Could you check a few things on this model? Use its own coordinates, in mm. A direction names the side the tool comes from. Coordinates: 2 decimals unless noted, no trailing zeros. Write each loop counter-clockwise with the first axis right and the second up, starting at its lowest first coordinate (ties: lowest second). Pieces come first, ordered by that corner, then holes.
```python
from build123d import *

# Parameters (mm, degrees)
F0_W      = 60
F0_H      = 15
F1_DEPTH  = 75
F2_DEPTH  = 15
F4_DEPTH  = 25
F6_DEPTH  = 40
F8_DEPTH  = 40
F10_DEPTH = 25


with BuildPart() as f1:
    # F0 (on Top) → F1 (new body)
    with BuildSketch(Plane.XY):
        with Locations((17.5909090042, 32.8136347234)):
            Rectangle(F0_W, F0_H)
    extrude(amount=F1_DEPTH)

    # F0 (on Top) → F2 (join)
    with BuildSketch(Plane.XY):
        with Locations((17.5909090042, 32.8136347234)):
            Rectangle(F0_W, F0_H)
        with BuildLine():
            Line((47.5909090042, 25.3136347234), (-12.4090909958, 25.3136347234))
            Line((-12.4090909958, 25.3136347234), (-12.4090909958, -29.6863652766))
            ThreePointArc((-12.4090909958, -29.6863652766), (17.5909090042, 0.3136347234), (47.5909090042, -29.6863652766))
            Line((47.5909090042, -29.6863652766), (47.5909090042, 25.3136347234))
        make_face()
        with BuildLine():
            ThreePointArc((47.5909090042, -29.6863652766), (17.5909090042, 0.3136347234), (-12.4090909958, -29.6863652766))
            Line((-12.4090909958, -29.6863652766), (47.5909090042, -29.6863652766))
        make_face()
        with BuildLine():
            Line((47.5909090042, -29.6863652766), (-12.4090909958, -29.6863652766))
            ThreePointArc((-12.4090909958, -29.6863652766), (17.5909090042, -59.6863652766), (47.5909090042, -29.6863652766))
        make_face()
    extrude(amount=F2_DEPTH)

    # F3 (on face) → F4 (cut)
    with BuildSketch(Plane.XY.offset(15)):
        with BuildLine():
            ThreePointArc((7.5909090042, -57.970636524), (17.5909090042, -59.6863652766), (27.5909090042, -57.970636524))
            Line((27.5909090042, -57.970636524), (27.5909090042, -29.6863652766))
            ThreePointArc((27.5909090042, -29.6863652766), (17.5909090042, -39.6863652766), (7.5909090042, -29.6863652766))
            Line((7.5909090042, -29.6863652766), (7.5909090042, -57.970636524))
        make_face()
        with BuildLine():
            ThreePointArc((7.5909090042, -29.6863652766), (17.5909090042, -39.6863652766), (27.5909090042, -29.6863652766))
            Line((27.5909090042, -29.6863652766), (17.5909090042, -29.6863652766))
            Line((17.5909090042, -29.6863652766), (7.5909090042, -29.6863652766))
        make_face()
        with BuildLine():
            Line((17.5909090042, -29.6863652766), (27.5909090042, -29.6863652766))
            ThreePointArc((27.5909090042, -29.6863652766), (17.5909090042, -19.6863652766), (7.5909090042, -29.6863652766))
            Line((7.5909090042, -29.6863652766), (17.5909090042, -29.6863652766))
        make_face()
    extrude(amount=-F4_DEPTH, mode=Mode.SUBTRACT)

    # F5 (on face) → F6 (join)
    with BuildSketch(Plane(origin=(0, 40.3136347234, 0), x_dir=(-1, 0, 0), z_dir=(0, 1, 0))):
        with BuildLine():
            Line((-42.2313958406, 75), (-47.5909090042, 75))
            ThreePointArc((-47.5909090042, 75), (-17.5909090042, 45), (12.4090909958, 75))
            Line((12.4090909958, 75), (-2.5909090042, 75))
            ThreePointArc((-2.5909090042, 75), (-17.5909090042, 60), (-32.5909090042, 75))
            Line((-32.5909090042, 75), (-42.2313958406, 75))
        make_face()
    extrude(amount=F6_DEPTH)

    # F7 (on face) → F8 (join)
    with BuildSketch(Plane(origin=(0, 40.3136347234, 0), x_dir=(-1, 0, 0), z_dir=(0, 1, 0))):
        with BuildLine():
            Line((-22.5909090042, 45.4196010845), (-22.5909090042, 0))
            Line((-22.5909090042, 0), (-12.5909090042, 0))
            Line((-12.5909090042, 0), (-12.5909090042, 45.4196010845))
            ThreePointArc((-12.5909090042, 45.4196010845), (-17.5909090042, 45), (-22.5909090042, 45.4196010845))
        make_face()
    extrude(amount=F8_DEPTH)

    # F9 (on face) → F10 (cut)
    with BuildSketch(Plane(origin=(12.5909090042, 0, 0), x_dir=(0, -1, 0), z_dir=(-1, 0, 0))):
        Polygon((-40.3136347234, 0), (-80.3136347234, 45.4196010845), (-80.3136347234, 0), align=None)
    extrude(amount=-F10_DEPTH, mode=Mode.SUBTRACT)


solid = f1.part
```
1. I want a section at A-A on y = 45.5. Please give me the cut outline in (x, z), plus the area to 3 significant figures.
Verdict:
outline: (-12.41, 75) arc R30 ccw to (12.59, 45.42) - (12.59, 5.89) - (22.59, 5.89) - (22.59, 45.42) arc R30 ccw to (47.59, 75) - (32.59, 75) arc R15 cw to (2.59, 75) - close
area: 1,450 mm2
2. For pin 1 (12 mm diameter, centred on x = 11, y = 22, fed in from -Z); pin 2 (12 mm diameter, centred on y = -47.5, z = 10, fed in from +X); pin 3 (20 mm diameter, centred on y = 69.5, z = 22, fed in from -X); pin 4 (12 mm diameter, centred on x = 9, z = 22, fed in from +Y), each with a flat end and sliding along its axis, tell me the tip position at first contact or that it passes through.
Verdict:
pin 1: stops at z = 0
pin 2: stops at x = 45.17
pin 3: stops at x = 12.59
pin 4: stops at y = 63.92
3. I want a section at C-C on z = 51. Please give me the cut outline in (x, y).
Verdict:
outline: (-12.41, 25.31) - (47.59, 25.31) - (47.59, 40.31) - (35.59, 40.31) - (35.59, 80.31) - (-0.41, 80.31) - (-0.41, 40.31) - (-12.41, 40.31) - close
4. I want a section at B-B on x = 5. Please give me the cut outline in (y, z).
Verdict:
outline: (-56.92, 0) - (40.31, 0) - (40.31, 47.77) - (80.31, 47.77) - (80.31, 66.85) - (40.31, 66.85) - (40.31, 75) - (25.31, 75) - (25.31, 15) - (-56.92, 15) - close
5. Please list where these lines run through material, in increasing order: line 1 along X through (y, z) = (-51, 5.5); line 2 along Y through (x, z) = (-9, 19.5); line 3 along X through (y, z) = (64, 36.5).
Verdict:
line 1: x = -3.52 to 7.59, 27.59 to 38.7
line 2: y = 25.31 to 40.31
line 3: x = 12.59 to 22.59
6. I want a section at D-D on y = -48. Please give me the cut outline in (x, z), plus the area to 3 significant figures.
Verdict:
outline: (-6.17, 0) - (7.59, 0) - (7.59, 15) - (-6.17, 15) - close; (27.59, 0) - (41.35, 0) - (41.35, 15) - (27.59, 15) - close
area: 413 mm2
7. If we mould it in two halves opening along X, with no side actions, what happens to faces 6 (the face through (17, -6, 15)), 7 (the face through (27.591, -44, 8)), 8 (the face through (-5.13, 60.03, 55.41)), 9 (the face through (41.936, -47.217, 7.395))? For each: pulls with the +X half, pulls with the -X half, needs draft (parallel to the pull), parting line crosses it, or undercut.
Verdict:
face 6: needs draft
face 7: undercut
face 8: pulls with the -X half
face 9: pulls with the +X half
8. On a 3-axis mill with a long thin cutter (end or side, diameter ignored), from which of +Z, -Z, +X, -X, +Y, -Y can I reach the whole of each face in a straight line? I mean faces 1 (the face through (7.591, -44, 8)), 2 (the face through (35, 40.314, 29)), 3 (the face through (17.52, 60.03, 22.39)), 4 (the face through (17, 25.314, 45)), 5 (the face through (17.261, 60.034, 60.004)). Say none if no direction works.
Verdict:
face 1: +Z, -Z, -Y
face 2: -Z, +X, +Y
face 3: -Z, +X, -X, +Y
face 4: +Z, +X, -X, -Y
face 5: +Z, +Y
